from build123d import *

# Parameters (mm, degrees)
F0_W   = 1.5191692636
F0_H   = 15.0828957558
F0_W_2 = 1.0024315159
F0_H_2 = 9.863063693


with BuildPart() as f1:
    # F0 (on Front) → F1 (revolve)
    with BuildSketch(Plane.XZ):
        Polygon((36.4248545221, 0), (21.3932929025, 50), (21.3932929025, 62.3753145337), (20.3490806933, 62.3753145337), (20.3490806933, 59.1916404665), (20.32, 59.1916404665), (20.32, 59.2419579625), (20.3073, 59.2419579625), (19.3048684841, 56.1876572669), (19.3048684841, 50), (30.9293307364, 11.333151716), (32.4485, 6.2798867857), (34.3364301037, 0), align=None)
        Polygon((32.4485, 0), (34.3364301037, 0), (32.4485, 6.2798867857), align=None)
        Polygon((32.4485, 0), (32.4485, 6.2798867857), (30.9293307364, 11.333151716), (30.9293307364, 0), align=None)
        with Locations((31.6889153682, -7.5414478779)):
            Rectangle(F0_W, F0_H)
        with Locations((19.806084242, 67.3068463802)):
            Rectangle(F0_W_2, F0_H_2)
        Polygon((20.3073, 59.2419579625), (20.3073, 62.3753145337), (19.3048684841, 62.3753145337), (19.3048684841, 56.1876572669), align=None)
    revolve(axis=Axis((0, 0, 25), (0, 0, 1)))


solid = f1.part
Can you work these out from the model? Positions are in its coordinate system, mm. A direction names the side the tool comes from. Round coordinates to 2 decimals unless told otherwise and drop trailing zeros. Write each loop counter-clockwise with the first axis right and the second up, starting at its lowest first coordinate (ties: lowest second). Pieces come first, ordered by that corner, then holes. Notation, with made-up numbers: (60.25, -28.5) -> (94.25, -28.5) arc R12 ccw to (94.25, -8.5) -> close; hole circle Ø8 at (-37, -23). An arc over 180 degrees is marked (long way). Use one line per item in the form item = value. Start each with the question number.
Q1. Imagine slicing it at D-D (z = 29.5). Please give me the cut outline in (x, y), then the cut area to 3 significant figures.
Q2. If I drill on probe 1 along Y at (x, z) = (0, 62.5); probe 2 along Y at (x, z) = (0, -2.25); probe 3 along X at (y, z) = (1, 59), over which ranges is the centre line in solid material (lowest first)? Write a range as [from, to].
Q3. I'm going to push flat-ended pins straight in: P1, Ø8, axis at x = 21.5, z = 35.5, coming from the +Y side; P2, Ø1.5, axis at y = 1.5, z = 15, coming from the +X side; P3, Ø1.5, axis at y = -5.5, z = 45.5, coming from the -X side. Where does each tip first touch, or does it pass through?
Q4. We'd pull the mould along Y, two halves only. Please class faces 1 (the face through (-7.034, -31.677, -7.436)), 2 (the face through (-4.185, -18.846, 61.275)), 3 (the face through (33, -3, 0)): +Y half, -Y half, draft (parallel to the pull), parting line (faces both ways), or undercut.
Q5. Which directions (+Z, -Z, +X, -X, +Y, -Y) give clear straight access to the entire face, cutting with the end or side of a thin tool? Please do faces 4 (the face through (29.5, 9.3, -2.1)), 5 (the face through (-7.4, -18, 72.238)), 6 (the face through (20.405, 6.426, 56.274)).
Q6. Imagine slicing it at C-C (z = 58). Please give me the cut outline in (x, y).
Worked out:
q1.outline = circle Ø55.11 at (0, 0); hole circle Ø50.94 at (0, 0)
q1.area = 348 mm^2
q2.probe_1 = [-20.31, -19.3], [19.3, 20.31]
q2.probe_2 = [-32.45, -30.93], [30.93, 32.45]
q2.probe_3 = [-21.37, -19.28], [19.28, 21.37]
q3.P1 = 19.24
q3.P2 = 32.11
q3.P3 = -22.36
q4.face_1 = parting line
q4.face_2 = undercut
q4.face_3 = draft
q5.face_4 = -Z
q5.face_5 = +Z, +X, -X, +Y, -Y
q5.face_6 = +Z
q6.outline = circle Ø42.79 at (0, 0); hole circle Ø38.61 at (0, 0)
